Verification items for this drawing (mm, ordinates from the low corner). A direction names the side the tool comes from. Give positions to 0.01 mm unless a question says otherwise; leave off trailing zeros. Order: outer loops, then holes, each group sorted by start corner. A loop starts at its lowest first (then second) coordinate and runs counter-clockwise, first axis right, second up. Notation, with made-up numbers: M 31.25,39.5 L 38.25,39.5 A11 ccw 38.25,43.5 Z; hole C 30.5,82 d3. An arc over 180 degrees is marked long. Answer as a JSON object with one key per item and string values.
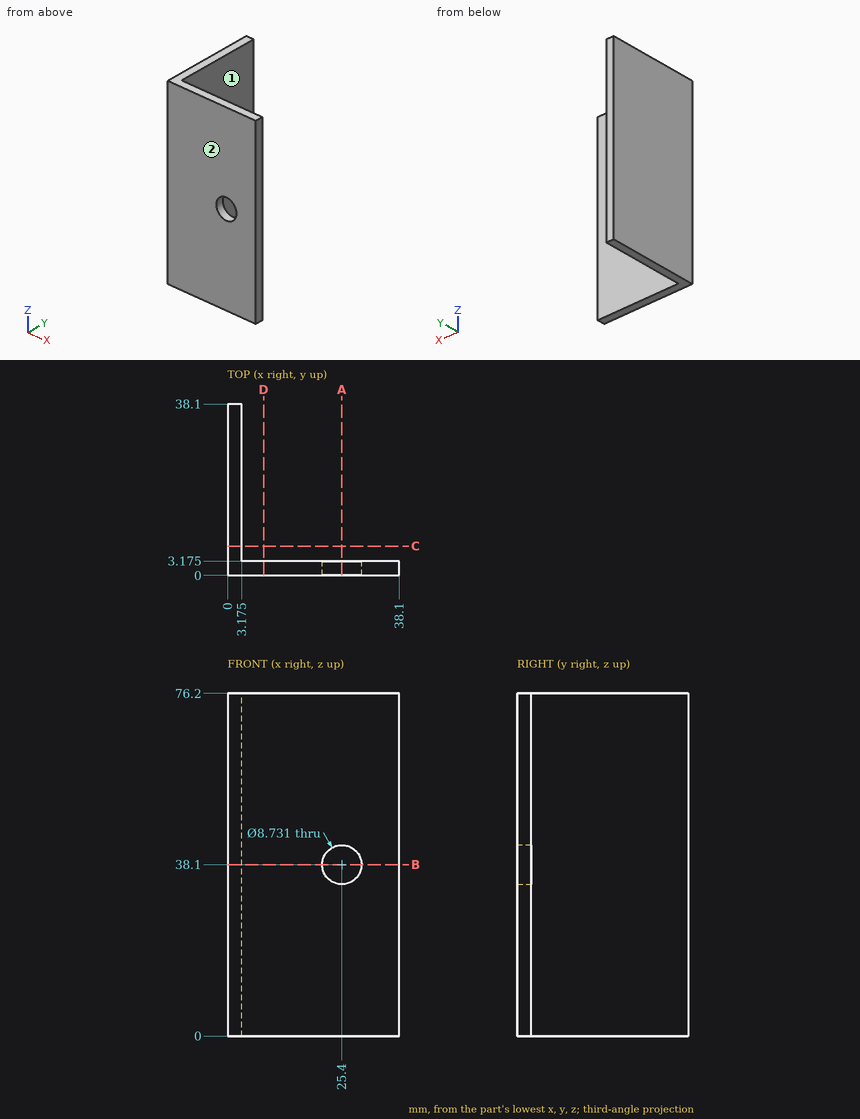
Q1. Section check A-A on x = 25.4. Record the cut outline in (y, z) (1 decimal), then the cut area to 3 significant figures.
Resolved:
{"outline": "M 0,0 L 3.2,0 L 3.2,33.7 L 0,33.7 Z; M 0,42.5 L 3.2,42.5 L 3.2,76.2 L 0,76.2 Z", "area": "214 mm²"}
Q2. Gauge pin test, flat ends, axial feed: pin 1 Ø12 at (x, z) = (19.5, 37) entering from +Y (3 decimals); pin 2 Ø12 at (x, y) = (32.5, 9.5) entering from +Z; pin 3 Ø10.5 at (y, z) = (20.5, 39.5) entering from +X (3 decimals). Record the tip position at first contact, or that the pin passes through.
Resolved:
{"pin 1": "stops at y = 3.175", "pin 2": "passes through", "pin 3": "stops at x = 3.175"}
Q3. Section check B-B on z = 38.1. Record the cut outline in (x, y) (1 decimal), then the cut area to 3 significant figures.
Resolved:
{"outline": "M 0,0 L 21,0 L 21,3.2 L 3.2,3.2 L 3.2,38.1 L 0,38.1 Z; M 29.8,0 L 38.1,0 L 38.1,3.2 L 29.8,3.2 Z", "area": "204 mm²"}
Q4. Material ranges on L1, parallel to Z at x = 25, y = 1; L2, parallel to X at y = 1.5, z = 38.1; L3, parallel to Y at x = 21.5, z = 4 (1 decimal), recorded low to high.
Resolved:
{"L1": "z = 0 to 33.75, 42.45 to 76.2", "L2": "x = 0 to 21.03, 29.77 to 38.1", "L3": "y = 0 to 3.2"}
Q5. Tool access check on the marked faces 1 and 2. Record the directions out of +Z, -Z, +X, -X, +Y, -Y that give a thin tool (end or side, any length) a straight path to the whole face; none if there is none.
Resolved:
{"face 1": "+Z, -Z, +X, +Y", "face 2": "+Z, -Z, +X, -X, -Y"}
Q6. Section check C-C on y = 6.5. Record the cut outline in (x, z) (1 decimal), then the cut area to 3 significant figures.
Resolved:
{"outline": "M 0,0 L 3.2,0 L 3.2,76.2 L 0,76.2 Z", "area": "242 mm²"}
